Here's the drawing with two shaded views (mm, measured from the low corner). I have some questions. Round coordinates to 2 decimals unless told otherwise and drop trailing zeros. Order: outer loops, then holes, each group sorted by start corner. A loop starts at its lowest first (then second) coordinate and runs counter-clockwise, first axis right, second up. Notation, with made-up numbers: (50.5, 15.25) - (81.5, 15.25) arc R35 ccw to (81.5, 48.25) - close; hole circle Ø6 at (-0.5, -22). An arc over 180 degrees is marked (long way). One line per item, written item: value.
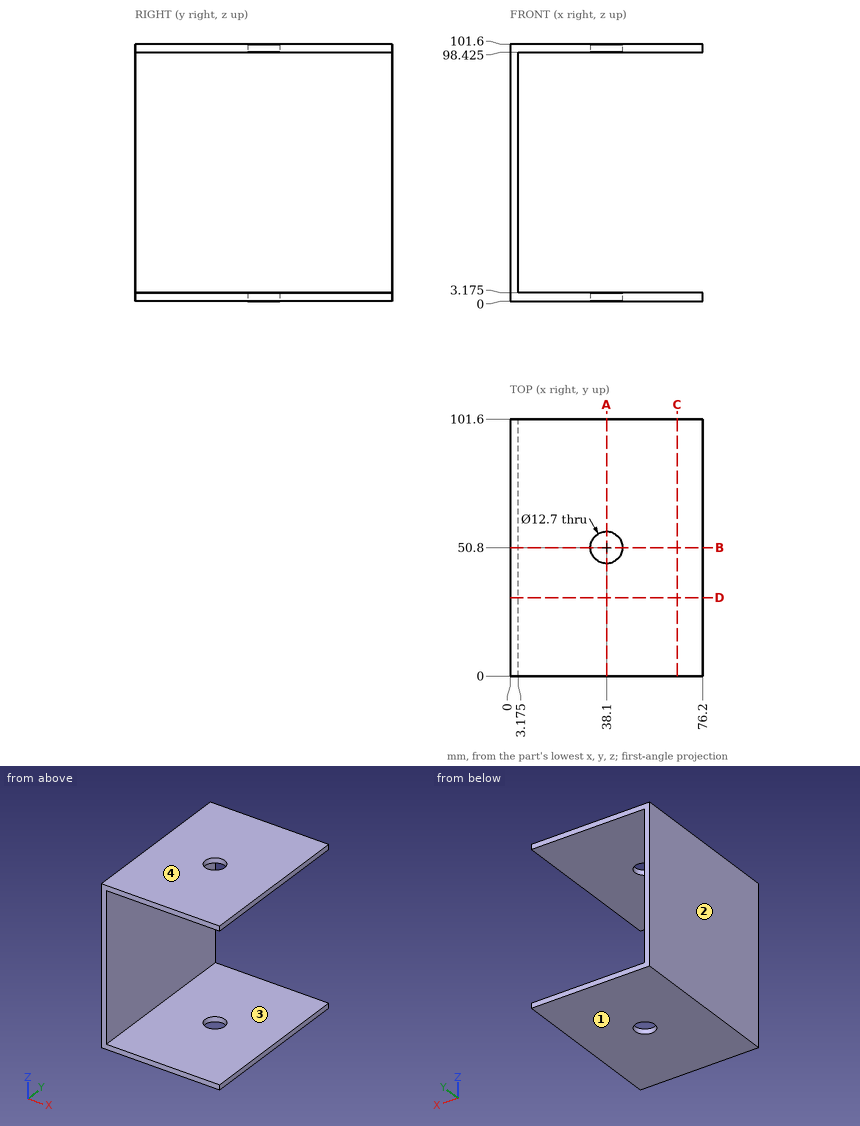
Q1. If we section it at C-C, the plane x = 66: Please give me the cut outline in (y, z) (3 decimals).
Results list:
outline: (0, 0) - (101.6, 0) - (101.6, 3.175) - (0, 3.175) - close; (0, 98.425) - (101.6, 98.425) - (101.6, 101.6) - (0, 101.6) - close
Q2. If I drill on line 1 along Z through (x, y) = (69, 87) (3 decimals); line 2 along Y through (x, z) = (38.1, 1.75); line 3 along X through (y, z) = (50.8, 1.2), over which ranges is the centre line in solid material (lowest first)?
Results list:
line 1: 0 to 3.175, 98.425 to 101.6
line 2: 0 to 44.45, 57.15 to 101.6
line 3: 0 to 31.75, 44.45 to 76.2
Q3. If we section it at D-D, the plane y = 31: Please give me the cut outline in (x, z) (3 decimals), then the cut area to 3 significant figures.
Results list:
outline: (0, 0) - (76.2, 0) - (76.2, 3.175) - (3.175, 3.175) - (3.175, 98.425) - (76.2, 98.425) - (76.2, 101.6) - (0, 101.6) - close
area: 786 mm²
Q4. If we section it at B-B, the plane y = 50.8: Please give me the cut outline in (x, z) (3 decimals).
Results list:
outline: (0, 0) - (31.75, 0) - (31.75, 3.175) - (3.175, 3.175) - (3.175, 98.425) - (31.75, 98.425) - (31.75, 101.6) - (0, 101.6) - close; (44.45, 0) - (76.2, 0) - (76.2, 3.175) - (44.45, 3.175) - close; (44.45, 98.425) - (76.2, 98.425) - (76.2, 101.6) - (44.45, 101.6) - close
Q5. Will these pins go through, and if not, where does the flat tip stop? pin 1 (8 mm diameter, centred on y = 23, z = 31, fed in from -X); pin 2 (11.5 mm diameter, centred on x = 38.1, y = 50.8, fed in from +Z).
Results list:
pin 1: x = 0
pin 2: through
Q6. We'd pull the mould along Z, two halves only. Please class the marked faces 1, 2, 3 and 4: released by +Z, released by -Z, zero draft, split by the parting line, or undercut.
Results list:
face 1: released by -Z
face 2: zero draft
face 3: undercut
face 4: released by +Z
Q7. If we section it at A-A, the plane x = 38.1: Please give me the cut outline in (y, z) (3 decimals), then the cut area to 3 significant figures.
Results list:
outline: (0, 0) - (44.45, 0) - (44.45, 3.175) - (0, 3.175) - close; (0, 98.425) - (44.45, 98.425) - (44.45, 101.6) - (0, 101.6) - close; (57.15, 0) - (101.6, 0) - (101.6, 3.175) - (57.15, 3.175) - close; (57.15, 98.425) - (101.6, 98.425) - (101.6, 101.6) - (57.15, 101.6) - close
area: 565 mm²
